Check sheet for the modelled part. Datum: model origin and axes. Units: mm. Face numbers are marked on the shaded views. A direction names the side the tool comes from. Give positions to 0.01 mm unless a question says otherwise; leave off trailing zeros. Loops run counter-clockwise (first coordinate to the right, second up) from the corner with the lowest first, then second, coordinate; pieces in that order, holes last. Notation, with made-up numbers: (33, 29.5) - (70, 29.5) arc R29 ccw to (70, 56.5) - close; hole circle Ø9 at (64.5, -10). An arc over 180 degrees is marked (long way). Use one line per item in the form item = value.
from build123d import *

# Parameters (mm, degrees)
SKETCH1_W           = 26.416
SKETCH1_H           = 31.75
BOSS_EXTRUDE1_DEPTH = 5.08
SKETCH2_W           = 16.51
SKETCH2_H           = 7.62
SKETCH2_W_2         = 3.81
CUT_EXTRUDE1_DEPTH  = 5.08
SKETCH3_W           = 19.05
SKETCH3_H           = 22.098
BOSS_EXTRUDE2_DEPTH = 26.416
BOSS_EXTRUDE3_DEPTH = 3.048
BOSS_EXTRUDE4_DEPTH = 3.048
BOSS_EXTRUDE5_DEPTH = 17.78
BOSS_EXTRUDE6_DEPTH = 17.78
SKETCH10_R          = 2.54
CUT_EXTRUDE3_DEPTH  = 17.78
SKETCH11_W          = 20.32
SKETCH11_H          = 30.981160888
CUT_EXTRUDE4_DEPTH  = 22.86
FILLET3_R           = 2.54
FILLET4_R           = 2.54
SKETCH12_W          = 26.416
SKETCH12_H          = 14.732
SKETCH12_R          = 2.54
BOSS_EXTRUDE7_DEPTH = 16.383
FILLET5_R           = 1.27
FILLET6_R           = 1.27


with BuildPart() as part:
    # Sketch1 → Boss-Extrude1 (new body)
    with BuildSketch(Plane(origin=(0, 0, 0), x_dir=(1, 0, 0), z_dir=(0, 1, 0))):
        with Locations((2.032, 9.525)):
            Rectangle(SKETCH1_W, SKETCH1_H)
        with BuildLine():
            ThreePointArc((5.244874103, -0.8509), (-1.524, 0.6731), (5.244874103, 2.1971))
            Line((5.244874103, 2.1971), (10.922, 2.1971))
            Line((10.922, 2.1971), (10.922, -0.8509))
            Line((10.922, -0.8509), (5.244874103, -0.8509))
        make_face(mode=Mode.SUBTRACT)
    extrude(amount=BOSS_EXTRUDE1_DEPTH)

    # Sketch2 → Cut-Extrude1 (cut)
    with BuildSketch(Plane(origin=(0, 5.08, 0), x_dir=(1, 0, 0), z_dir=(0, 1, 0))):
        with Locations((0.127, 14.1351)):
            Rectangle(SKETCH2_W, SKETCH2_H)
        with Locations((10.287, 14.1351)):
            Rectangle(SKETCH2_W_2, SKETCH2_H)
    extrude(amount=-CUT_EXTRUDE1_DEPTH, mode=Mode.SUBTRACT)

    # Sketch3 → Boss-Extrude2 (add)
    with BuildSketch(Plane.ZY.offset(11.176)):
        with Locations((-15.875, -11.049)):
            Rectangle(SKETCH3_W, SKETCH3_H)
        Polygon((-25.4, -22.098), (-6.35, -22.098), (-25.4, -30.981160888), align=None)
    extrude(amount=-BOSS_EXTRUDE2_DEPTH)

    # Sketch6 → Boss-Extrude3 (add)
    with BuildSketch(Plane.ZY.offset(11.176)):
        Polygon((6.35, 0), (-6.35, -11.049), (-6.35, 0), align=None)
    extrude(amount=-BOSS_EXTRUDE3_DEPTH)

    # Sketch7 → Boss-Extrude4 (add)
    with BuildSketch(Plane(origin=(15.24, 0, 0), x_dir=(0, 0, -1), z_dir=(1, 0, 0))):
        Polygon((-6.35, 0), (6.35, -11.049), (6.35, 0), align=None)
    extrude(amount=-BOSS_EXTRUDE4_DEPTH)

    # Sketch8 → Boss-Extrude5 (add)
    with BuildSketch(Plane(origin=(15.24, 0, 0), x_dir=(0, 0, -1), z_dir=(1, 0, 0))):
        Polygon((6.35, -22.098), (25.4, -30.981160888), (25.4, -27.171160888), (6.35, -18.288), align=None)
    extrude(amount=BOSS_EXTRUDE5_DEPTH)

    # Sketch9 → Boss-Extrude6 (add)
    with BuildSketch(Plane.ZY.offset(11.176)):
        Polygon((-6.35, -22.098), (-25.4, -30.981160888), (-25.4, -27.171160888), (-6.35, -18.288), align=None)
    extrude(amount=BOSS_EXTRUDE6_DEPTH)

    # Sketch10 → Cut-Extrude3 (cut)
    with BuildSketch(Plane(origin=(0, -12.589458796, 5.870561049), x_dir=(1, 0, 0), z_dir=(0, 0.9063077870366494, -0.42261826174070083))):
        with Locations(Location((24.13, 23.993528218, 0), (0, 0, 270))):
            Circle(SKETCH10_R)
        with Locations(Location((-20.066, 23.993528218, 0), (0, 0, 270))):
            Circle(SKETCH10_R)
    extrude(amount=-CUT_EXTRUDE3_DEPTH, mode=Mode.SUBTRACT)

    # Sketch11 → Cut-Extrude4 (cut)
    with BuildSketch(Plane(origin=(0, 0, -25.4), x_dir=(-1, 0, 0), z_dir=(0, 0, -1))):
        with Locations((-2.032, -15.490580444)):
            Rectangle(SKETCH11_W, SKETCH11_H)
    extrude(amount=-CUT_EXTRUDE4_DEPTH, mode=Mode.SUBTRACT)

    # Fillet3
    # the kernel refuses this fillet: 2.54 mm, written as the material it adds along each edge
    with BuildSketch(Plane(origin=(-8.128, 0, -25.4), x_dir=(0, -1, 0), z_dir=(0, 0, 1)), Plane(origin=(12.192, 0, -25.4), x_dir=(-1, 0, 0), z_dir=(0, 0, 1))) as fillet3_piece_1:
        with BuildLine():
            CenterArc((FILLET3_R, FILLET3_R), FILLET3_R, 180, 90)
            Line((0, FILLET3_R), (0, 0))
            Line((0, 0), (FILLET3_R, 0))
        make_face()
    extrude(amount=7.4549)
    with BuildSketch(Plane(origin=(-8.128, 0, -10.3251), x_dir=(1, 0, 0), z_dir=(0, 0, 1))) as fillet3_piece_2_section:
        with BuildLine():
            CenterArc((FILLET3_R, -FILLET3_R), FILLET3_R, 90, 90)
            Line((0, -FILLET3_R), (0, 0))
            Line((0, 0), (FILLET3_R, 0))
        make_face()
    fillet3_piece_2 = extrude(amount=16.6751, mode=Mode.PRIVATE)
    fillet3_piece_2 = split(fillet3_piece_2, bisect_by=Plane(origin=(-7.540337897, -4.52533198, 1.148468989), z_dir=(0, 0.7544430785777146, -0.6563654783626119)), keep=Keep.TOP, mode=Mode.PRIVATE)
    add(fillet3_piece_2)
    with BuildSketch(Plane(origin=(12.192, 0, 6.35), x_dir=(-1, 0, 0), z_dir=(0, 0, -1))) as fillet3_piece_3_section:
        with BuildLine():
            CenterArc((FILLET3_R, -FILLET3_R), FILLET3_R, 90, 90)
            Line((0, -FILLET3_R), (0, 0))
            Line((0, 0), (FILLET3_R, 0))
        make_face()
    fillet3_piece_3 = extrude(amount=16.6751, mode=Mode.PRIVATE)
    fillet3_piece_3 = split(fillet3_piece_3, bisect_by=Plane(origin=(10.504295152, -0.059519406, 0.8509), z_dir=(0, 0, 1)), keep=Keep.TOP, mode=Mode.PRIVATE)
    fillet3_piece_3 = split(fillet3_piece_3, bisect_by=Plane(origin=(10.922, -0.059519406, 3.561570264), z_dir=(-1, 0, 0)), keep=Keep.TOP, mode=Mode.PRIVATE)
    fillet3_piece_3 = split(fillet3_piece_3, bisect_by=Plane(origin=(10.504295152, -1.406445505, 4.733395971), z_dir=(0, 0.7544430785777146, -0.6563654783626119)), keep=Keep.TOP, mode=Mode.PRIVATE)
    add(fillet3_piece_3)
    with BuildSketch(Plane(origin=(12.192, 0, 6.35), x_dir=(-1, 0, 0), z_dir=(0, 0, -1))) as fillet3_piece_4_section:
        with BuildLine():
            CenterArc((FILLET3_R, -FILLET3_R), FILLET3_R, 90, 90)
            Line((0, -FILLET3_R), (0, 0))
            Line((0, 0), (FILLET3_R, 0))
        make_face()
    fillet3_piece_4 = extrude(amount=16.6751, mode=Mode.PRIVATE)
    fillet3_piece_4 = split(fillet3_piece_4, bisect_by=Plane(origin=(11.748492429, -0.576014265, 0.8509), z_dir=(0, 0, 1)), keep=Keep.TOP, mode=Mode.PRIVATE)
    fillet3_piece_4 = split(fillet3_piece_4, bisect_by=Plane(origin=(10.922, -0.576014265, 3.268620732), z_dir=(1, 0, 0)), keep=Keep.TOP, mode=Mode.PRIVATE)
    fillet3_piece_4 = split(fillet3_piece_4, bisect_by=Plane(origin=(11.748492429, -1.774025363, 4.310890388), z_dir=(0, 0.7544430785777146, -0.6563654783626119)), keep=Keep.TOP, mode=Mode.PRIVATE)
    add(fillet3_piece_4)
    with BuildSketch(Plane(origin=(12.192, 0, 6.35), x_dir=(-1, 0, 0), z_dir=(0, 0, -1))) as fillet3_piece_5_section:
        with BuildLine():
            CenterArc((FILLET3_R, -FILLET3_R), FILLET3_R, 90, 90)
            Line((0, -FILLET3_R), (0, 0))
            Line((0, 0), (FILLET3_R, 0))
        make_face()
    fillet3_piece_5 = extrude(amount=16.6751, mode=Mode.PRIVATE)
    fillet3_piece_5 = split(fillet3_piece_5, bisect_by=Plane(origin=(11.774444919, -0.648004952, 0.8509), z_dir=(0, 0, -1)), keep=Keep.TOP, mode=Mode.PRIVATE)
    fillet3_piece_5 = split(fillet3_piece_5, bisect_by=Plane(origin=(10.922, -0.648004952, -0.6731), z_dir=(1, 0, 0)), keep=Keep.TOP, mode=Mode.PRIVATE)
    fillet3_piece_5 = split(fillet3_piece_5, bisect_by=Plane(origin=(11.774444919, -0.648004952, -2.1971), z_dir=(0, 0, 1)), keep=Keep.TOP, mode=Mode.PRIVATE)
    add(fillet3_piece_5)
    with BuildSketch(Plane(origin=(12.192, 0, 6.35), x_dir=(-1, 0, 0), z_dir=(0, 0, -1))) as fillet3_piece_6_section:
        with BuildLine():
            CenterArc((FILLET3_R, -FILLET3_R), FILLET3_R, 90, 90)
            Line((0, -FILLET3_R), (0, 0))
            Line((0, 0), (FILLET3_R, 0))
        make_face()
    fillet3_piece_6 = extrude(amount=16.6751, mode=Mode.PRIVATE)
    fillet3_piece_6 = split(fillet3_piece_6, bisect_by=Plane(origin=(10.922, -0.060981289, -6.2611), z_dir=(-1, 0, 0)), keep=Keep.TOP, mode=Mode.PRIVATE)
    fillet3_piece_6 = split(fillet3_piece_6, bisect_by=Plane(origin=(10.507343007, -0.060981289, -2.1971), z_dir=(0, 0, -1)), keep=Keep.TOP, mode=Mode.PRIVATE)
    add(fillet3_piece_6)
    with BuildSketch(Plane(origin=(12.192, 0, 6.35), x_dir=(-1, 0, 0), z_dir=(0, 0, -1))) as fillet3_piece_7_section:
        with BuildLine():
            CenterArc((FILLET3_R, -FILLET3_R), FILLET3_R, 90, 90)
            Line((0, -FILLET3_R), (0, 0))
            Line((0, 0), (FILLET3_R, 0))
        make_face()
    fillet3_piece_7 = extrude(amount=16.6751, mode=Mode.PRIVATE)
    fillet3_piece_7 = split(fillet3_piece_7, bisect_by=Plane(origin=(10.922, -0.648004952, -6.2611), z_dir=(1, 0, 0)), keep=Keep.TOP, mode=Mode.PRIVATE)
    fillet3_piece_7 = split(fillet3_piece_7, bisect_by=Plane(origin=(11.774444919, -0.648004952, -2.1971), z_dir=(0, 0, -1)), keep=Keep.TOP, mode=Mode.PRIVATE)
    add(fillet3_piece_7)
    with BuildSketch(Plane(origin=(15.24, -29.85478685, -31.155054448), x_dir=(1, 0, 0), z_dir=(0, 0.42261826174070066, 0.9063077870366494))) as fillet3_piece_8_section:
        with BuildLine():
            CenterArc((FILLET3_R, FILLET3_R), FILLET3_R, 180, 90)
            Line((0, FILLET3_R), (0, 0))
            Line((0, 0), (FILLET3_R, 0))
        make_face()
    fillet3_piece_8 = extrude(amount=33.719349356, mode=Mode.PRIVATE)
    fillet3_piece_8 = split(fillet3_piece_8, bisect_by=Plane(origin=(15.81504359, -22.095090044, -25.4), z_dir=(0, 0, 1)), keep=Keep.TOP, mode=Mode.PRIVATE)
    fillet3_piece_8 = split(fillet3_piece_8, bisect_by=Plane(origin=(15.81504359, -22.095090044, -6.35), z_dir=(0, 0, -1)), keep=Keep.TOP, mode=Mode.PRIVATE)
    add(fillet3_piece_8)
    with BuildSketch(Plane(origin=(-11.176, -29.85478685, -31.155054448), x_dir=(0, 0.9063077870366492, -0.4226182617407009), z_dir=(0, 0.4226182617407009, 0.9063077870366493))) as fillet3_piece_9_section:
        with BuildLine():
            CenterArc((FILLET3_R, FILLET3_R), FILLET3_R, 180, 90)
            Line((0, FILLET3_R), (0, 0))
            Line((0, 0), (FILLET3_R, 0))
        make_face()
    fillet3_piece_9 = extrude(amount=33.719349356, mode=Mode.PRIVATE)
    fillet3_piece_9 = split(fillet3_piece_9, bisect_by=Plane(origin=(-11.75104359, -22.095090044, -25.4), z_dir=(0, 0, 1)), keep=Keep.TOP, mode=Mode.PRIVATE)
    fillet3_piece_9 = split(fillet3_piece_9, bisect_by=Plane(origin=(-11.75104359, -22.095090044, -6.35), z_dir=(0, 0, -1)), keep=Keep.TOP, mode=Mode.PRIVATE)
    add(fillet3_piece_9)

    # Fillet4
    fillet4_edges = [part.edges().sort_by_distance(p)[0] for p in [
        (-9.652, -11.049, -6.35),
        (13.716, -11.049, -6.35),
    ]]
    fillet(fillet4_edges, radius=FILLET4_R)

    # Sketch12 → Boss-Extrude7 (add)
    with BuildSketch(Plane(origin=(0, 5.08, 0), x_dir=(1, 0, 0), z_dir=(0, 1, 0))):
        with Locations((2.032, 32.766)):
            Rectangle(SKETCH12_W, SKETCH12_H)
        with Locations(Location((2.032, 32.766, 0), (0, 0, 270))):
            Circle(SKETCH12_R, mode=Mode.SUBTRACT)
    extrude(amount=-BOSS_EXTRUDE7_DEPTH)

    # Fillet5
    fillet5_edges = [part.edges().sort_by_distance(p)[0] for p in [
        (12.192, -6.9215, -25.4),
        (2.032, 0, -25.4),
        (-7.384051224, -0.743948776, -25.4),
        (11.448051224, -0.743948776, -25.4),
        (-8.128, -6.9215, -25.4),
    ]]
    fillet(fillet5_edges, radius=FILLET5_R)

    # Fillet6
    fillet6_edges = [part.edges().sort_by_distance(p)[0] for p in [
        (13.716, -11.303, -25.4),
        (-9.652, -11.303, -25.4),
    ]]
    fillet(fillet6_edges, radius=FILLET6_R)


solid = part.part
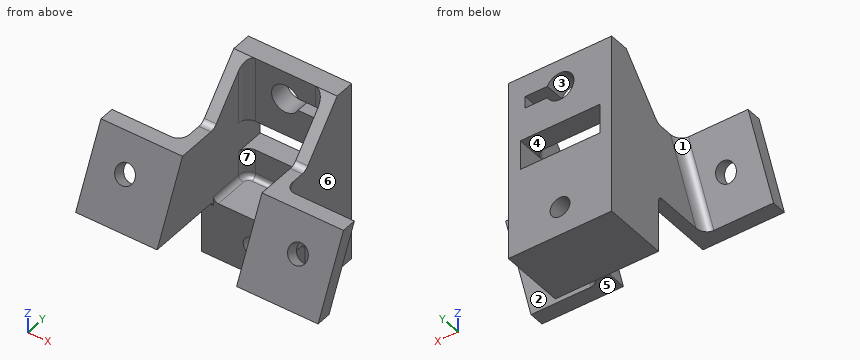
Item 1: Section check B-B on z = -1. Record the boundary of the cut face in (x, y).
Answer block:
outline = (-11.18, -6.39) - (-8.13, -6.39) - (-8.13, -2.54) arc R2.54 cw to (-5.59, 0) - (-1.51, 0) - (-1.51, 5.08) - (-11.18, 5.08) - close; (10.92, -0.34) arc R2.54 cw to (12.19, -2.54) - (12.19, -6.39) - (15.24, -6.39) - (15.24, 5.08) - (10.92, 5.08) - close
Item 2: Gauge pin test, flat ends, axial feed: P1, Ø3, axis at x = 3.5, y = -5.5, coming from the +Z side; P2, Ø6, axis at y = -11, z = -21, coming from the +X side; P3, Ø5, axis at x = 12, z = -8, coming from the -Y side; P4, Ø6, axis at x = -1.5, y = -14.5, coming from the +Z side. Record the tip position at first contact, or that the pin passes through.
Answer block:
P1 = -25.4
P2 = 15.24
P3 = -24.03
P4 = through
Item 3: Section check A-A on y = -14. Record the boundary of the cut face in (x, z).
Answer block:
outline = (-11.18, -25.4) - (-8.13, -25.4) - (-8.13, -6.35) - (-11.18, -6.35) - close; (12.19, -25.4) - (15.24, -25.4) - (15.24, -6.35) - (12.19, -6.35) - close
Item 4: Access from +Z, -Z, +X, -X, +Y, -Y to the whole of each face (thin tool, end or side, straight path). Record for the marked faces 4, 5, 6 and 7.
Answer block:
face_4 = +Y, -Y
face_5 = -Z, +X, -X, -Y
face_6 = -Z, +X, +Y
face_7 = +Z, -Y
Item 5: Thickness scan on L1, parallel to X at y = -18.5, z = -14; L2, parallel to Y at x = 9, z = -35.5; L3, parallel to Z at x = 2.5, y = -10. Record the ranges inside material, lowest first.
Answer block:
L1 = -11.18 to -8.13, 12.19 to 15.24
L2 = -11.3 to 5.08
L3 = -40.13 to -35.26, -30.27 to -25.4
Item 6: Section check D-D on x = -19. Record the boundary of the cut face in (y, z).
Answer block:
outline = (-30.98, -25.4) - (-27.17, -25.4) - (-23.7, -17.96) - (-26.83, -16.51) - close; (-24.88, -12.33) - (-21.76, -13.79) - (-18.29, -6.35) - (-22.1, -6.35) - close
Item 7: Section check C-C on y = -6. Record the boundary of the cut face in (x, z), then the cut area to 3 significant figures.
Answer block:
outline = (-11.18, -40.13) - (15.24, -40.13) - (15.24, -0.55) - (12.19, -0.55) - (12.19, -24.13) arc R1.27 cw to (10.92, -25.4) - (-6.86, -25.4) arc R1.27 cw to (-8.13, -24.13) - (-8.13, -0.55) - (-11.18, -0.55) - close; hole circle Ø5.08 at (2.03, -32.77)
area = 521 mm2
Item 8: Mould release check, pull along X, two halves, no side actions. Record for the marked faces 1, 2 and 3: released by +X, released by -X, zero draft, split by the parting line, or undercut.
Answer block:
face_1 = released by -X
face_2 = zero draft
face_3 = undercut
